```python
from build123d import *

# Parameters (mm, degrees)
F0_W      = 635
F0_H      = 762
F1_DEPTH  = 12.7
F1_FACE_W = 635
F1_FACE_H = 762
F2_DEPTH  = 12.7
F3_W      = 12.7
F3_H      = 406.4
F4_DEPTH  = 101.6
F5_W      = 12.7
F5_H      = 406.4
F6_DEPTH  = 101.6
F8_DEPTH  = 12.7
F9_W      = 635
F9_H      = 127
F10_DEPTH = 12.7


with BuildPart() as f1:
    # F0 (on Front) → F1 (new body)
    with BuildSketch(Plane.XZ):
        with Locations((8.002397, -204.813847)):
            Rectangle(F0_W, F0_H)
    extrude(amount=F1_DEPTH)

    # F1_face (on face) → F2 (join)
    with BuildSketch(Plane(origin=(8.002397, -12.7, -204.813847), x_dir=(1, 0, 0), z_dir=(0, -1, 0))):
        Rectangle(F1_FACE_W, F1_FACE_H)
    extrude(amount=F2_DEPTH)

    # F3 (on face) → F4 (join)
    with BuildSketch(Plane.XZ.offset(25.4)):
        with Locations((-303.147603, -382.613847)):
            Rectangle(F3_W, F3_H)
    extrude(amount=F4_DEPTH)

    # F5 (on face) → F6 (join)
    with BuildSketch(Plane.XZ.offset(25.4)):
        with Locations((319.152397, -382.613847)):
            Rectangle(F5_W, F5_H)
    extrude(amount=F6_DEPTH)

    # F7 (on face) → F8 (join)
    with BuildSketch(Plane.XZ.offset(127)):
        Polygon((328.198969, -179.413847), (-309.497603, -179.413847), (-309.497603, -585.813847), (328.198969, -586.074769), align=None)
    extrude(amount=F8_DEPTH)

    # F9 (on face) → F10 (join)
    with BuildSketch(Plane(origin=(0, 0, -585.813847), x_dir=(1, 0, 0), z_dir=(0, 0, -1))):
        with Locations((8.002397, 63.5)):
            Rectangle(F9_W, F9_H)
    extrude(amount=F10_DEPTH)


solid = f1.part
```
Can you work these out from the model? Positions are in its coordinate system, mm. A direction names the side the tool comes from. Give positions to 0.01 mm unless a question says otherwise; leave off trailing zeros. Order: outer loops, then holes, each group sorted by start corner. A loop starts at its lowest first (then second) coordinate and runs counter-clockwise, first axis right, second up. Notation, with made-up numbers: M 42,42.25 L 76,42.25 A14 cw 76,59.25 Z; hole C 65.5,9 d4. An arc over 180 degrees is marked long. One line per item, written item: value.
1) For P1, Ø6.5, axis at x = 34, z = -593, coming from the -Y side; P2, Ø6, axis at x = -194, z = 97, coming from the -Y side; P3, Ø1.5, axis at x = -2.5, z = -248, coming from the +Y side; P4, Ø6.5, axis at x = 93, y = -136, coming from the -Z side, each with a flat end and sliding along its axis, tell me the tip position at first contact or that it passes through.
Answer sheet:
P1: stops at y = -127
P2: stops at y = -25.4
P3: stops at y = 0
P4: stops at z = -585.98
2) We'd pull the mould along X, two halves only. Please class faces 1 (the face through (4, -127, -380)), 2 (the face through (-309.498, -53, -292)), 3 (the face through (5, -139.7, -380)): released by +X, released by -X, zero draft, split by the parting line, or undercut.
Answer sheet:
face 1: undercut
face 2: released by -X
face 3: zero draft
3) I want a section at D-D, the plane z = 126. List the corners of the cut face in (x, y) for me.
Answer sheet:
outline: M -309.5,-25.4 L 325.5,-25.4 L 325.5,0 L -309.5,0 Z
4) On a 3-axis mill with a long thin cutter (end or side, diameter ignored), from which of +Z, -Z, +X, -X, +Y, -Y can I reach the whole of each face in a straight line? I mean faces 4 (the face through (4, 0, -206)), 5 (the face through (325.502, -48, -292)), 6 (the face through (4, -77, -585.814)), 7 (the face through (82, -129, -179.414)). Say none if no direction works.
Answer sheet:
face 4: +Z, -Z, +X, -X, +Y
face 5: +Z, -Z, +X, +Y
face 6: +Z
face 7: +Z, +X, -X, -Y
5) Please list where these lines run through material, in increasing order: line 1 along X through (y, z) = (-73.5, -312); line 2 along Y through (x, z) = (-258, -509); line 3 along Y through (x, z) = (-9.5, 46).
Answer sheet:
line 1: x = -309.5 to -296.8, 312.8 to 325.5
line 2: y = -139.7 to -127, -25.4 to 0
line 3: y = -25.4 to 0
6) I want a section at A-A, the plane z = -405. List the corners of the cut face in (x, y) for me.
Answer sheet:
outline: M -309.5,-139.7 L 328.2,-139.7 L 328.2,-127 L 325.5,-127 L 325.5,0 L -309.5,0 Z; hole M -296.8,-127 L 312.8,-127 L 312.8,-25.4 L -296.8,-25.4 Z
7) I want a section at B-B, the plane x = -112. List the corners of the cut face in (y, z) for me.
Answer sheet:
outline: M -139.7,-585.89 L -127,-585.89 L -127,-598.51 L 0,-598.51 L 0,176.19 L -25.4,176.19 L -25.4,-585.81 L -127,-585.81 L -127,-179.41 L -139.7,-179.41 Z
8) I want a section at C-C, the plane y = -39.5. List the corners of the cut face in (x, z) for me.
Answer sheet:
outline: M -309.5,-598.51 L 325.5,-598.51 L 325.5,-179.41 L 312.8,-179.41 L 312.8,-585.81 L -296.8,-585.81 L -296.8,-179.41 L -309.5,-179.41 Z
